The figure shows three views and two pictorial views of one solid part (mm, origin at its lowest corner). Answer the questions. Coordinates: 2 decimals unless noted, no trailing zeros. Loops run counter-clockwise (first coordinate to the right, second up) from the corner with the lowest first, then second, coordinate; pieces in that order, holes last. Notation, with made-up numbers: (21, -7.75) - (59, -7.75) arc R8 cw to (59, -1.75) - close; hole circle Ø8 at (-2, 65.5). An arc over 180 degrees is marked (long way). Write each question's results on one line, items separated by ' | '. Start each with the question number.
Item 1: For a pull along Y with two mould halves and no side action, classify the marked faces 1, 2 and 3 as +Y half, -Y half, draft (parallel to the pull), parting line (faces both ways), or undercut.
Item 2: Section B-B, the plane y = 7.62 is taken. Count the separate pieces of the cut face and the enclosed holes in it, plus the area to 3 significant figures.
Item 3: Section A-A, the plane x = 8.89 is taken. Write down the section's boundary in (y, z), plus the area to 3 significant figures.
Item 4: Consider probe 1 along Y at (x, z) = (42, 2.5); probe 2 along X at (y, z) = (9, 13); probe 3 along X at (y, z) = (12.25, 10). Determine where each line is inside the solid, lowest interval first. Write a range as [from, to].
Item 5: Section C-C, the plane z = 16.5 is taken. Write down the section's boundary in (x, y), plus the area to 3 significant figures.
Item 6: Section D-D, the plane z = 10.25 is taken. Write down the section's boundary in (x, y), plus the area to 3 significant figures.
Item 7: Each of these flat-tipped pins is pushed along its axis until it touches: pin 1 Ø6 at (x, y) = (41.91, 7.62) entering from +Z; pin 2 Ø7.5 at (x, y) = (8.89, 7.62) entering from +Z. Where does it stop, or does it pass through?
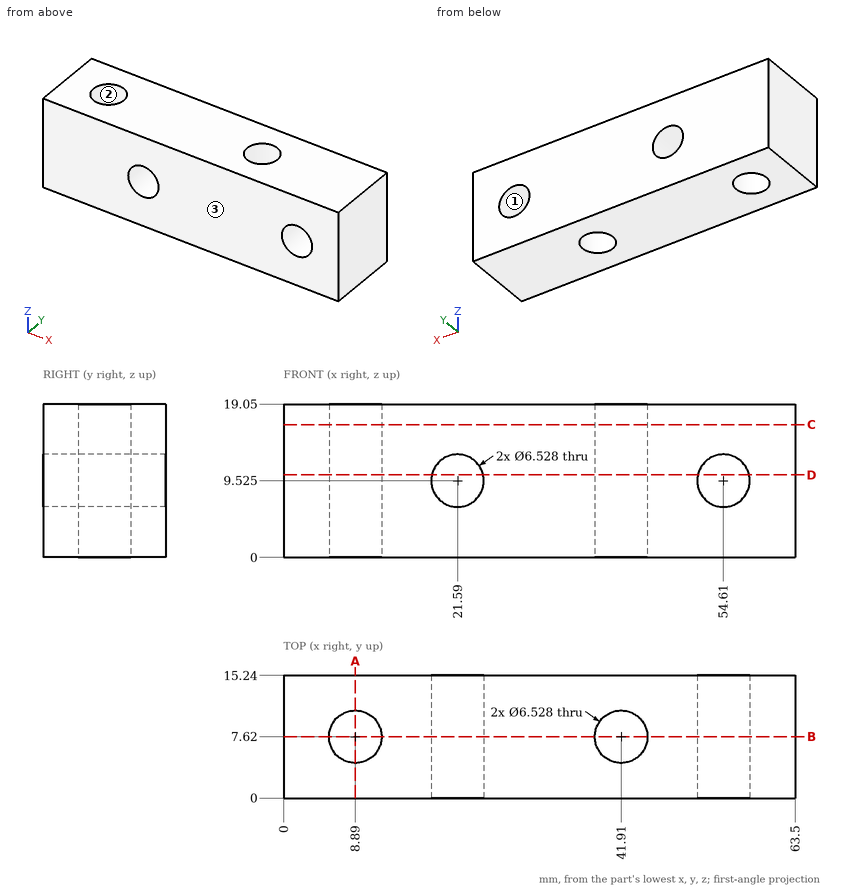
Answer key:
1) face 1: draft | face 2: undercut | face 3: -Y half
2) separate pieces: 3 | enclosed holes: 2 | area: 894 mm^2
3) outline: (0, 0) - (4.36, 0) - (4.36, 19.05) - (0, 19.05) - close; (10.88, 0) - (15.24, 0) - (15.24, 19.05) - (10.88, 19.05) - close | area: 166 mm^2
4) probe 1: y = [0, 4.36], [10.88, 15.24] | probe 2: x = [0, 5.93], [11.85, 38.95], [44.87, 63.5] | probe 3: x = [0, 18.36], [24.82, 51.38], [57.84, 63.5]
5) outline: (0, 0) - (63.5, 0) - (63.5, 15.24) - (0, 15.24) - close; hole circle Ø6.53 at (8.89, 7.62); hole circle Ø6.53 at (41.91, 7.62) | area: 901 mm^2
6) outline: (0, 0) - (18.41, 0) - (18.41, 15.24) - (0, 15.24) - close; (24.77, 0) - (51.43, 0) - (51.43, 15.24) - (24.77, 15.24) - close; (57.79, 0) - (63.5, 0) - (63.5, 15.24) - (57.79, 15.24) - close; hole circle Ø6.53 at (8.89, 7.62); hole circle Ø6.53 at (41.91, 7.62) | area: 707 mm^2
7) pin 1: passes through | pin 2: stops at z = 19.05
